Part model, mm, in its own coordinate system. A direction names the side the tool comes from. Give positions to 0.01 mm unless a question says otherwise; leave off trailing zeros. Write each loop counter-clockwise with the first axis right and the second up, starting at its lowest first coordinate (ties: lowest second). Pieces come first, ordered by that corner, then holes. Notation, with made-up numbers: M -9.75,-7.75 L 11.25,-7.75 A29 cw 11.25,28.25 Z; hole C -0.5,7.5 d11. An arc over 180 degrees is marked long. Use a Markdown table: item, result. Add a question column.
from build123d import *

# Parameters (mm, degrees)
F0_W          = 53.975
F0_H          = 31.75
F1_DEPTH      = 6.35
F2_R          = 15.875
F3_DEPTH      = 6.35
F3_DEPTH_BACK = 6.35
F4_R          = 9.525
F5_DEPTH      = 25.4
F6_W          = 31.75
F6_H          = 6.35
F6_R          = 9.525
F7_DEPTH      = 9.525
F8_R          = 9.525
F9_DEPTH      = 9.652
F9_DEPTH_BACK = 9.525
F12_DEPTH     = 3.175
F13_R         = 2.54
F14_DEPTH     = 19.051
F15_R         = 1.7272
F16_DEPTH     = 31.751
F17_W         = 22.1996
F17_H         = 7.874
F18_DEPTH     = 8.001
F19_R         = 0.762
F24_R         = 1.7272
F25_DEPTH     = 12.7
F27_R         = 1.7272
F28_DEPTH     = 12.7


with BuildPart() as f1:
    # F0 (on Top) → F1 (new body)
    with BuildSketch(Plane.XY):
        with Locations((-26.9875, -15.875)):
            Rectangle(F0_W, F0_H)
    extrude(amount=F1_DEPTH)

    # F2 (on face) → F3 (join, two sides)
    with BuildSketch(Plane.XY.offset(6.35)) as f3_sk:
        with Locations((-53.975, -15.875)):
            Circle(F2_R)
    extrude(amount=F3_DEPTH)
    extrude(f3_sk.sketch, amount=-F3_DEPTH_BACK)

    # F4 (on face) → F5 (cut)
    with BuildSketch(Plane.XY.offset(12.7)):
        with Locations((-53.975, -15.875)):
            Circle(F4_R)
    extrude(amount=-F5_DEPTH, mode=Mode.SUBTRACT)

    # F6 (on face) → F7 (join)
    with BuildSketch(Plane.YZ):
        with BuildLine():
            Line((0, 6.35), (0, 25.4))
            ThreePointArc((0, 25.4), (-15.875, 9.525), (-31.75, 25.4))
            Line((-31.75, 25.4), (-31.75, 6.35))
            Line((-31.75, 6.35), (0, 6.35))
        make_face()
        with Locations((-15.875, 3.175)):
            Rectangle(F6_W, F6_H)
        with BuildLine():
            ThreePointArc((-31.75, 25.4), (-15.875, 9.525), (0, 25.4))
            ThreePointArc((0, 25.4), (-15.875, 41.275), (-31.75, 25.4))
        make_face()
        with Locations((-15.875, 25.4)):
            Circle(F6_R, mode=Mode.SUBTRACT)
    extrude(amount=-F7_DEPTH)

    # F8 (on face) → F9 (join, two sides)
    with BuildSketch(Plane.YZ) as f9_sk:
        with Locations((-15.875, 25.4)):
            Circle(F8_R)
    extrude(amount=F9_DEPTH)
    extrude(f9_sk.sketch, amount=-F9_DEPTH_BACK)

    # F11 (on offset) → F12 (join, symmetric)
    with BuildSketch(Plane.XZ.offset(15.875)):
        Polygon((-9.525, 6.35), (-9.525, 25.4), (-34.3816611394, 11.049), (-34.3816611394, 12.7), (-38.9536611394, 12.7), (-38.9536611394, 6.35), align=None)
    extrude(amount=F12_DEPTH, both=True)

    # F13 (on face) → F14 (cut, through all)
    with BuildSketch(Plane.XZ.offset(19.05)):
        with Locations((-35.9090883884, 13.0784250415)):
            Circle(F13_R)
    extrude(amount=-F14_DEPTH, mode=Mode.SUBTRACT)

    # F15 (on face) → F16 (cut, through all)
    with BuildSketch(Plane.XZ.offset(31.75)):
        with Locations((-3.175, 8.763)):
            Circle(F15_R)
    extrude(amount=-F16_DEPTH, mode=Mode.SUBTRACT)

    # F17 (on face) → F18 (cut)
    with BuildSketch(Plane.YZ):
        with Locations((-15.875, 8.763)):
            Rectangle(F17_W, F17_H)
    extrude(amount=-F18_DEPTH, mode=Mode.SUBTRACT)

    # F19
    f19_edges = [f1.edges().sort_by_distance(p)[0] for p in [
        (-4.0005, -4.7752, 4.826),
        (-8.001, -15.875, 4.826),
        (-4.0005, -26.9748, 4.826),
        (-8.001, -15.875, 12.7),
        (-4.0005, -4.7752, 12.7),
        (-4.0005, -26.9748, 12.7),
        (-8.001, -26.9748, 8.763),
        (-8.001, -4.7752, 8.763),
        (-9.525, -19.05, 15.875),
        (-9.525, -12.7, 15.875),
    ]]
    fillet(f19_edges, radius=F19_R)

    # F24 (on offset) → F25 (cut)
    with BuildSketch(Plane(origin=(-47.3526280605, -47.3526280605, 0), x_dir=(0.7071067812, -0.7071067812, 0), z_dir=(-0.7071067812, -0.7071067812, 0))):
        with Locations((-26.9995890558, 7.874)):
            Circle(F24_R)
    extrude(amount=-F25_DEPTH, mode=Mode.SUBTRACT)

    # F27 (on offset) → F28 (cut)
    with BuildSketch(Plane(origin=(-31.4692606164, 31.4692606164, 0), x_dir=(-0.7071067812, -0.7071067812, 0), z_dir=(-0.7071067812, 0.7071067812, 0))):
        with Locations((49.6344417334, 7.874)):
            Circle(F27_R)
    extrude(amount=-F28_DEPTH, mode=Mode.SUBTRACT)


solid = f1.part
1. Tool access for faces 5 (the flat face through (-4, -16, 12.7)), 6 (the flat face through (-27, -25, 6.35)), 7 (the flat face through (-61, -9, 12.7)): list every direction of +Z, -Z, +X, -X, +Y, -Y with a clear straight run to the whole face (end or side of a thin tool).
2. Cut at C-C (z = 37). Write the cut outline in (x, y) (3 decimals), then the cut area to 3 significant figures.
3. Drill centre lines: probe 1 along X at (y, z) = (-13, 11); probe 2 along Z at (x, y) = (-29.5, -9); probe 3 along X at (y, z) = (-9.5, 33) (3 decimals). Where is each one in solid material? Low to high. Write a range as [from, to].
4. Flat gauge pins, fed straight in: pin 1 (6 mm diameter, centred on x = -49, z = 7.5, fed in from +Y); pin 2 (10 mm diameter, centred on x = -21.5, z = 16, fed in from +Y); pin 3 (1.5 mm diameter, centred on x = -53.5, y = -5.5, fed in from +Z); pin 4 (6.5 mm diameter, centred on x = -29, y = -25.5, fed in from +Z). Where does each tip first touch, or does it go through?
5. Cut at B-B (z = 20). Write the cut outline in (x, y) (3 decimals), then the cut area to 3 significant figures.
6. Mould opens along Y. For faces 1 (the flat face through (-21, -19.05, 14)), 2 (the cylindrical face through (-45.176, -19.523, 6.439)), 3 (the flat face through (-27, -6, 6.35)), 4 (the flat face through (-21, -12.7, 14)) say: released by +Y, released by -Y, zero draft, split by the parting line, or undercut.
7. Cut at A-A (x = -12). Write the cut outline in (y, z), then the cut area to 3 significant figures.
A:
| question | item | result |
|---|---|---|
| 1 | face 5 | +X |
| 1 | face 6 | +Z, -Y |
| 1 | face 7 | +Z, -X, +Y, -Y |
| 2 | outline | M -9.525,-26.713 L 0,-26.713 L 0,-5.037 L -9.525,-5.037 Z |
| 2 | area | 206 mm² |
| 3 | probe 1 | x = [-69.59, -63.06], [-44.89, -37.37], [-34.45, -8] |
| 3 | probe 2 | z = [0, 6.35] |
| 3 | probe 3 | x = [-9.525, 0] |
| 4 | pin 1 | stops at y = 0 |
| 4 | pin 2 | stops at y = -12.7 |
| 4 | pin 3 | stops at z = 12.7 |
| 4 | pin 4 | stops at z = 6.35 |
| 5 | outline | M -18.878,-19.05 L -10.287,-19.05 A0.762 cw -9.525,-19.812 L -9.525,-31.75 L 0,-31.75 L 0,-23.721 L 9.652,-23.721 L 9.652,-8.029 L 0,-8.029 L 0,0 L -9.525,0 L -9.525,-11.938 A0.762 cw -10.287,-12.7 L -18.878,-12.7 Z |
| 5 | area | 514 mm² |
| 6 | face 1 | released by -Y |
| 6 | face 2 | undercut |
| 6 | face 3 | zero draft |
| 6 | face 4 | released by +Y |
| 7 | outline | M -31.75,0 L 0,0 L 0,6.35 L -12.7,6.35 L -12.7,23.97 L -19.05,23.97 L -19.05,6.35 L -31.75,6.35 Z |
| 7 | area | 314 mm² |
